For this review, take the finished solid that the model builds, in its own axes (mm). A direction names the side the tool comes from. Round coordinates to 2 decimals unless told otherwise and drop trailing zeros. Write each loop counter-clockwise with the first axis right and the second up, starting at its lowest first coordinate (ties: lowest second). Pieces come first, ordered by that corner, then holes. Notation, with made-up numbers: (32, -11) -> (44, -11) arc R31 cw to (44, 27) -> close; hole circle Ø2 at (63.5, 10). An arc over 180 degrees is marked (long way). Answer in a Markdown table with one row per item.
from build123d import *

# Parameters (mm, degrees)
PAD009_DEPTH    = 2.8
FILLET004_R     = 0.4
POCKET014_DEPTH = 2.801
SKETCH028_R     = 8.5
POCKET017_DEPTH = 2.801


with BuildPart() as part:
    # Sketch009 → Pad009 (new body)
    with BuildSketch(Plane.XZ.offset(60.5)):
        with BuildLine():
            Line((37.8, 3.2), (37.8, 0.4))
            Line((37.8, 0.4), (23.8, 0.4))
            ThreePointArc((23.8, 0.4), (23.4, 0), (23.8, -0.4))
            Line((23.8, -0.4), (37.8, -0.4))
            Line((37.8, -0.4), (37.8, -33.8))
            Line((37.8, -33.8), (23.8, -33.8))
            ThreePointArc((23.8, -33.8), (23.4, -34.2), (23.8, -34.6))
            Line((23.8, -34.6), (37.8, -34.6))
            Line((37.8, -34.6), (37.8, -37.4))
            Line((37.8, -37.4), (35.8, -38.4))
            Line((35.8, -38.4), (35.8, -37.4))
            Line((35.8, -37.4), (33, -37.4))
            Line((33, -37.4), (33, -39.4))
            Line((33, -39.4), (25.535898, -37.4))
            Line((25.535898, -37.4), (-25.535898, -37.4))
            Line((-25.535898, -37.4), (-33, -39.4))
            Line((-33, -39.4), (-33, -37.4))
            Line((-33, -37.4), (-35.8, -37.4))
            Line((-35.8, -38.4), (-35.8, -37.4))
            Line((-37.8, -37.4), (-35.8, -38.4))
            Line((-37.8, -37.4), (-37.8, -34.6))
            Line((-37.8, -34.6), (-23.8, -34.6))
            ThreePointArc((-23.8, -34.6), (-23.4, -34.2), (-23.8, -33.8))
            Line((-23.8, -33.8), (-37.8, -33.8))
            Line((-37.8, -33.8), (-37.8, -0.4))
            Line((-37.8, -0.4), (-23.8, -0.4))
            ThreePointArc((-23.8, -0.4), (-23.4, 0), (-23.8, 0.4))
            Line((-23.8, 0.4), (-37.8, 0.4))
            Line((-37.8, 0.4), (-37.8, 3.2))
            Line((-37.8, 3.2), (-35.8, 4.2))
            Line((-35.8, 4.2), (-35.8, 3.2))
            Line((-35.8, 3.2), (-33, 3.2))
            Line((-33, 3.2), (-33, 5.2))
            Line((-33, 5.2), (-25.535898, 3.2))
            Line((-25.535898, 3.2), (25.535898, 3.2))
            Line((25.535898, 3.2), (33, 5.2))
            Line((33, 5.2), (33, 3.2))
            Line((33, 3.2), (35.8, 3.2))
            Line((35.8, 3.2), (35.8, 4.2))
            Line((37.8, 3.2), (35.8, 4.2))
        make_face()
    extrude(amount=-PAD009_DEPTH)

    # Fillet004
    fillet004_edges = [part.edges().sort_by_distance(p)[0] for p in [
        (37.8, -59.1, -0.4),
        (37.8, -59.1, 0.4),
        (37.8, -59.1, 3.2),
        (25.535898, -59.1, 3.2),
        (-25.535898, -59.1, 3.2),
        (-37.8, -59.1, 3.2),
        (-37.8, -59.1, 0.4),
        (-37.8, -59.1, -0.4),
        (-37.8, -59.1, -33.8),
        (-37.8, -59.1, -34.6),
        (-37.8, -59.1, -37.4),
        (-25.535898, -59.1, -37.4),
        (25.535898, -59.1, -37.4),
        (37.8, -59.1, -37.4),
        (37.8, -59.1, -34.6),
        (37.8, -59.1, -33.8),
    ]]
    fillet(fillet004_edges, radius=FILLET004_R)

    # Sketch025 → Pocket014 (cut, through all)
    with BuildSketch(Plane.XZ.offset(60.5)):
        with BuildLine():
            ThreePointArc((-24, -4.49), (-24.755, -5.245), (-24, -6))
            Line((-24, -6), (-12, -6))
            ThreePointArc((-12, -6), (-11.245, -5.245), (-12, -4.49))
            Line((-24, -4.49), (-12, -4.49))
        make_face()
        with BuildLine():
            ThreePointArc((12, -4.49), (11.245, -5.245), (12, -6))
            Line((12, -6), (24, -6))
            ThreePointArc((24, -6), (24.755, -5.245), (24, -4.49))
            Line((12, -4.49), (24, -4.49))
        make_face()
    extrude(amount=-POCKET014_DEPTH, mode=Mode.SUBTRACT)

    # Sketch028 → Pocket017 (cut, through all)
    with BuildSketch(Plane.XZ.offset(60.5)):
        with Locations((-12.8, -24.1)):
            Circle(SKETCH028_R)
        with Locations((12.8, -24.1)):
            Circle(SKETCH028_R)
        with BuildLine():
            ThreePointArc((-2.85, -29.7), (-5.35, -32.2), (-2.85, -34.7))
            Line((-2.85, -34.7), (2.85, -34.7))
            ThreePointArc((2.85, -34.7), (5.35, -32.2), (2.85, -29.7))
            Line((-2.85, -29.7), (2.85, -29.7))
        make_face()
    extrude(amount=-POCKET017_DEPTH, mode=Mode.SUBTRACT)


solid = part.part
1) For faces 1 (the flat face through (-31, -59, -0.4)), 2 (the flat face through (31, -59, -33.8)), 3 (the flat face through (0, -59, -29.7)), 4 (the flat face through (-34, -59, 3.2)), 5 (the flat face through (36.7, -59.12, 3.75)), list the 3-axis set-ups (+Z, -Z, +X, -X, +Y, -Y) from which the entire face can be reached by the end or side of a thin tool; tool diameter is ignored.
Solved:
| item | result |
|---|---|
| face 1 | -X, +Y, -Y |
| face 2 | +X, +Y, -Y |
| face 3 | +Y, -Y |
| face 4 | +Z, +Y, -Y |
| face 5 | +Z, +X, +Y, -Y |
2) Consider section C-C on y = -59.4. State how many separate pieces and enclosed holes the cut face has, then the cut area to 3 significant figures.
Solved:
| item | result |
|---|---|
| separate pieces | 1 |
| enclosed holes | 5 |
| area | 2,520 mm² |
3) For line 1 (X direction, y = -59.5, z = -24.5); line 2 (Z direction, x = 12.8, y = -59.05); line 3 (Z direction, x = 33.5, y = -59.3), list the stretches that pass through material, from the lowest coordinate up. Write a range as [from, to].
Solved:
| item | result |
|---|---|
| line 1 | [-37.8, -21.29], [-4.31, 4.31], [21.29, 37.8] |
| line 2 | [-37.4, -32.6], [-15.6, -6], [-4.49, 3.2] |
| line 3 | [-37.4, -34.6], [-33.8, -0.4], [0.4, 3.2] |
4) Mouldability with a two-part tool opening along X and no side actions: class faces 6 (the flat face through (-36.7, -59.12, 3.75)), 7 (the cylindrical face through (-8.23, -59.12, -16.933)), 8 (the flat face through (-31, -59, 0.4)) as pulls with the +X half, pulls with the -X half, needs draft (parallel to the pull), parting line crosses it, or undercut.
Solved:
| item | result |
|---|---|
| face 6 | pulls with the -X half |
| face 7 | undercut |
| face 8 | needs draft |
5) Consider section A-A on z = -24.1. State the section outline as (x, y) points, then the cut area to 3 significant figures.
Solved:
| item | result |
|---|---|
| outline | (-37.8, -60.5) -> (-21.3, -60.5) -> (-21.3, -57.7) -> (-37.8, -57.7) -> close; (-4.3, -60.5) -> (4.3, -60.5) -> (4.3, -57.7) -> (-4.3, -57.7) -> close; (21.3, -60.5) -> (37.8, -60.5) -> (37.8, -57.7) -> (21.3, -57.7) -> close |
| area | 116 mm² |
6) Clearance check with flat-ended pins moving along their axes: pin 1 Ø0.8 at (x, y) = (-28, -59.5) entering from -Z; pin 2 Ø1 at (x, y) = (7.5, -58.5) entering from +Z; pin 3 Ø0.5 at (y, z) = (-59, 4) entering from -X; pin 4 Ø2 at (x, z) = (5.5, -21.5) entering from +Y. State where each tip first meets the part, or that it passes through.
Solved:
| item | result |
|---|---|
| pin 1 | z = -38.17 |
| pin 2 | z = 3.2 |
| pin 3 | x = -36.7 |
| pin 4 | y = -57.7 |
7) Consider section B-B on x = -12.8. State the section outline as (y, z) points, then the cut area to 3 significant figures.
Solved:
| item | result |
|---|---|
| outline | (-60.5, -37.4) -> (-57.7, -37.4) -> (-57.7, -32.6) -> (-60.5, -32.6) -> close; (-60.5, -15.6) -> (-57.7, -15.6) -> (-57.7, -6) -> (-60.5, -6) -> close; (-60.5, -4.49) -> (-57.7, -4.49) -> (-57.7, 3.2) -> (-60.5, 3.2) -> close |
| area | 61.9 mm² |
